Geometry: final body of the model. Coordinates: model frame, mm. A direction names the side the tool comes from. Coordinates: 2 decimals unless noted, no trailing zeros. Order: outer loops, then holes, each group sorted by start corner. A loop starts at its lowest first (then second) coordinate and runs counter-clockwise, first axis right, second up. Notation, with made-up numbers: (57.25, 5.5) -> (97.25, 5.5) arc R27 ccw to (97.25, 36.5) -> close; hole circle Ø6 at (73, 75). An arc over 180 degrees is marked (long way). Use one line per item in the form item = value.
```python
from build123d import *

# Parameters (mm, degrees)
SKETCH2_W           = 60
SKETCH2_H           = 60
SKETCH2_W_2         = 40
SKETCH2_H_2         = 50
BOSS_EXTRUDE2_DEPTH = 23
SKETCH3_W           = 3
SKETCH3_H           = 18
CUT_EXTRUDE1_DEPTH  = 88.914731416


with BuildPart() as part:
    # Sketch2 → Boss-Extrude2 (new body)
    with BuildSketch(Plane(origin=(0, 0, 0), x_dir=(1, 0, 0), z_dir=(0, 1, 0))):
        with Locations((30, 30)):
            Rectangle(SKETCH2_W, SKETCH2_H)
        with Locations((30, 30)):
            Rectangle(SKETCH2_W_2, SKETCH2_H_2, mode=Mode.SUBTRACT)
    extrude(amount=BOSS_EXTRUDE2_DEPTH)

    # Sketch3 → Cut-Extrude1 (cut, through all)
    with BuildSketch(Plane.ZY):
        with Locations((-36, 14)):
            Rectangle(SKETCH3_W, SKETCH3_H)
        with Locations((-24, 14)):
            Rectangle(SKETCH3_W, SKETCH3_H)
    extrude(amount=-CUT_EXTRUDE1_DEPTH, mode=Mode.SUBTRACT)


solid = part.part
```
1) Material intervals for probe 1 along Z at (x, y) = (4.5, 20.5); probe 2 along Z at (x, y) = (31.5, 4.5); probe 3 along X at (y, z) = (2.5, -47), sorted ascending. Write a range as from..to.
Results found:
probe_1 = -60..-37.5, -34.5..-25.5, -22.5..0
probe_2 = -60..-55, -5..0
probe_3 = 0..10, 50..60
2) Access query for faces 4 (the flat face through (23, 23, -4)), 5 (the flat face through (10, 11, -30)), 6 (the flat face through (55, 14, -22.5)). Directions: +Z, -Z, +X, -X, +Y, -Y. A direction counts if a zero-diameter tool reaches every point of the face in a straight line with its end or side. Return the directions, or none.
Results found:
face_4 = +Z, -Z, +X, -X, +Y
face_5 = +Y, -Y
face_6 = +X, -X, +Y
3) Section C-C, the plane x = 13. Output: boundary loops of the cut face in (y, z), and give its area (3 significant figures).
Results found:
outline = (0, -60) -> (23, -60) -> (23, -55) -> (0, -55) -> close; (0, -5) -> (23, -5) -> (23, 0) -> (0, 0) -> close
area = 230 mm2
4) Pull-direction query (Z, two-part tool) for faces 1 (the flat face through (60, 11, -30)), 2 (the flat face through (55, 5, -24)), 3 (the flat face through (30, 11, 0)); classes: released by +Z, released by -Z, zero draft, split by the parting line, or undercut.
Results found:
face_1 = zero draft
face_2 = undercut
face_3 = released by +Z
5) Section A-A, the plane y = 21. Output: boundary loops of the cut face in (x, z), and give its area (3 significant figures).
Results found:
outline = (0, -60) -> (60, -60) -> (60, -37.5) -> (50, -37.5) -> (50, -55) -> (10, -55) -> (10, -37.5) -> (0, -37.5) -> close; (0, -34.5) -> (10, -34.5) -> (10, -25.5) -> (0, -25.5) -> close; (0, -22.5) -> (10, -22.5) -> (10, -5) -> (50, -5) -> (50, -22.5) -> (60, -22.5) -> (60, 0) -> (0, 0) -> close; (50, -34.5) -> (60, -34.5) -> (60, -25.5) -> (50, -25.5) -> close
area = 1,480 mm2
6) Contact query for a flat-ended pin moving along its axis: P1, Ø0.9, axis at x = 7, z = -35.5, coming from the +Y side. Output: stop coordinate, or through.
Results found:
P1 = 5
7) Section B-B, the plane z = -27. Output: boundary loops of the cut face in (x, y).
Results found:
outline = (0, 0) -> (10, 0) -> (10, 23) -> (0, 23) -> close; (50, 0) -> (60, 0) -> (60, 23) -> (50, 23) -> close
